from build123d import *

# Parameters (mm, degrees)
SKETCH1_W           = 19
SKETCH1_H           = 25.42
BOSS_EXTRUDE2_DEPTH = 10
FILLET1_R           = 3
SKETCH3_W           = 19.1
SKETCH3_H           = 2.2
CUT_EXTRUDE2_DEPTH  = 115.44
SKETCH4_R           = 9.475
SKETCH4_R_2         = 4.5
SKETCH4_R_3         = 6.33
SKETCH4_R_4         = 3.55
SKETCH4_R_5         = 1.25
CUT_EXTRUDE3_DEPTH  = 11
SKETCH5_W           = 42.44
SKETCH5_H           = 2.2
CUT_EXTRUDE4_DEPTH  = 90.1
SKETCH6_W           = 39.39
SKETCH6_H           = 25.42
CUT_EXTRUDE5_DEPTH  = 3.5
FILLET2_R           = 2
CUT_EXTRUDE6_DEPTH  = 6.5
CUT_EXTRUDE7_DEPTH  = 4.5


with BuildPart() as part:
    # Sketch1 → Boss-Extrude2 (new body)
    with BuildSketch(Plane(origin=(0, 0, 0), x_dir=(1, 0, 0), z_dir=(0, 1, 0))):
        Polygon((54.1, 18.1), (54.1, 0), (22.15, -56.030772795), (-22.15, -56.030772795), (-54.1, 0), (-54.1, 18.89218031), (-15.415468147, 58.409227205), (10.334531853, 58.409227205), align=None)
        with Locations((0, 7.599227205)):
            Rectangle(SKETCH1_W, SKETCH1_H, mode=Mode.SUBTRACT)
    extrude(amount=BOSS_EXTRUDE2_DEPTH)

    # Fillet1
    fillet1_edges = [part.edges().sort_by_distance(p)[0] for p in [
        (-9.5, 5, -20.309227205),
        (-9.5, 5, 5.110772795),
        (9.5, 5, 5.110772795),
        (9.5, 5, -20.309227205),
    ]]
    fillet(fillet1_edges, radius=FILLET1_R)

    # Sketch3 → Cut-Extrude2 (cut, through all)
    with BuildSketch(Plane(origin=(0, 0, -58.409227205), x_dir=(-1, 0, 0), z_dir=(0, 0, -1))):
        with Locations((44.55, 1.1)):
            Rectangle(SKETCH3_W, SKETCH3_H)
    extrude(amount=-CUT_EXTRUDE2_DEPTH, mode=Mode.SUBTRACT)

    # Sketch4 → Cut-Extrude3 (cut, through all)
    with BuildSketch(Plane(origin=(0, 10, 0), x_dir=(1, 0, 0), z_dir=(0, 1, 0))):
        with Locations((-3.065, 45.734227205)):
            Circle(SKETCH4_R)
        with Locations((14.065, -23.816239571)):
            Circle(SKETCH4_R_2)
        with Locations((-5.105, -23.816239571)):
            Circle(SKETCH4_R_2)
        with Locations((4.48, -43.150772795)):
            Circle(SKETCH4_R_2)
        with Locations((38.535, 4.609227205)):
            Circle(SKETCH4_R_3)
        with Locations((14.45, 15.849227205)):
            Circle(SKETCH4_R_4)
        with Locations((14.45, -0.650772795)):
            Circle(SKETCH4_R_4)
        with Locations((-14.45, -0.650772795)):
            Circle(SKETCH4_R_4)
        with Locations((-14.45, 15.849227205)):
            Circle(SKETCH4_R_4)
        with Locations((-50.45, 14.379227205)):
            Circle(SKETCH4_R_5)
    extrude(amount=-CUT_EXTRUDE3_DEPTH, mode=Mode.SUBTRACT)

    # Sketch5 → Cut-Extrude4 (cut, through all)
    with BuildSketch(Plane.ZY.offset(35)):
        with Locations((34.810772795, 1.1)):
            Rectangle(SKETCH5_W, SKETCH5_H)
    extrude(amount=-CUT_EXTRUDE4_DEPTH, mode=Mode.SUBTRACT)

    # Sketch6 → Cut-Extrude5 (cut)
    with BuildSketch(Plane.XZ):
        with Locations((0, -7.599227205)):
            Rectangle(SKETCH6_W, SKETCH6_H)
    extrude(amount=-CUT_EXTRUDE5_DEPTH, mode=Mode.SUBTRACT)

    # Fillet2
    fillet2_edges = [part.edges().sort_by_distance(p)[0] for p in [
        (19.695, 1.75, 5.110772795),
        (19.695, 1.75, -20.309227205),
        (-19.695, 1.75, -20.309227205),
        (-19.695, 1.75, 5.110772795),
    ]]
    fillet(fillet2_edges, radius=FILLET2_R)

    # Sketch4_3 → Cut-Extrude6 (cut)
    with BuildSketch(Plane(origin=(0, 10, 0), x_dir=(1, 0, 0), z_dir=(0, 1, 0))):
        with BuildLine():
            Line((-50, 8.869227205), (-50, 4.289227205))
            ThreePointArc((-50, 4.289227205), (-44.53, -1.180772795), (-39.06, 4.289227205))
            Line((-39.06, 4.289227205), (-39.06, 8.869227205))
            ThreePointArc((-39.06, 8.869227205), (-44.53, 14.339227205), (-50, 8.869227205))
        make_face()
    extrude(amount=-CUT_EXTRUDE6_DEPTH, mode=Mode.SUBTRACT)

    # Sketch7 → Cut-Extrude7 (cut, through all)
    with BuildSketch(Plane(origin=(0, 3.5, 0), x_dir=(-1, 0, 0), z_dir=(0, 1, 0))):
        with BuildLine():
            Line((41.28, -8.869227205), (41.28, -4.289227205))
            ThreePointArc((41.28, -4.289227205), (44.53, -1.039227205), (47.78, -4.289227205))
            Line((47.78, -4.289227205), (47.78, -8.869227205))
            ThreePointArc((47.78, -8.869227205), (44.53, -12.119227205), (41.28, -8.869227205))
        make_face()
    extrude(amount=-CUT_EXTRUDE7_DEPTH, mode=Mode.SUBTRACT)


solid = part.part
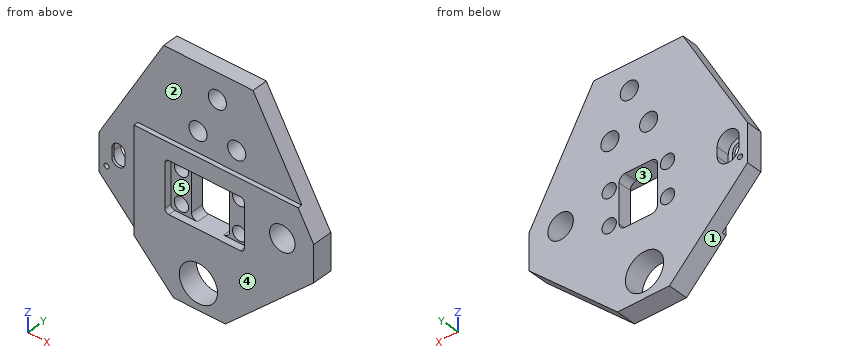
Could you check a few things on this model? Use its own coordinates, in mm. Face numbers are marked on the shaded views. A direction names the side the tool comes from. Round coordinates to 2 decimals unless told otherwise and drop trailing zeros. Write each loop counter-clockwise with the first axis right and the second up, starting at its lowest first coordinate (ties: lowest second). Pieces come first, ordered by that corner, then holes. Notation, with made-up numbers: (44.5, 56.5) -> (74.5, 56.5) arc R26 cw to (74.5, 73.5) -> close; hole circle Ø4 at (75.25, 5.25). An arc over 180 degrees is marked (long way). Use a Markdown table: item, result.
1. Which directions (+Z, -Z, +X, -X, +Y, -Y) give clear straight access to the entire face, cutting with the end or side of a thin tool? Please do the marked faces 4 and 5.
Answer key:
| item | result |
|---|---|
| face 4 | +Z, -Z, +X, -X, -Y |
| face 5 | -Y |
2. Please list where these lines run through material, in increasing order: probe 1 along Z at (x, y) = (-14.45, 6.25); probe 2 along Z at (x, y) = (1, 5.25); probe 3 along Y at (x, z) = (-42.5, -14).
Answer key:
| item | result |
|---|---|
| probe 1 | z = -58.41 to -19.4, -12.3 to -2.9, 4.2 to 56.03 |
| probe 2 | z = -58.41 to -54.29, -37.18 to -20.31, 5.11 to 40.3, 46 to 56.03 |
| probe 3 | y = 2.2 to 10 |
3. If we section it at C-C (x = -44.53): List the corners of the cut face in (y, z) for me, then the cut area to 3 significant figures.
Answer key:
| item | result |
|---|---|
| outline | (2.2, -28.67) -> (10, -28.67) -> (10, -14.34) -> (3.5, -14.34) -> (3.5, -12.12) -> (2.2, -12.12) -> close; (2.2, -1.04) -> (3.5, -1.04) -> (3.5, 1.18) -> (10, 1.18) -> (10, 16.78) -> (2.2, 16.78) -> close |
| area | 239 mm^2 |
4. For pin 1 Ø2 at (y, z) = (2.5, -26.5) entering from +X; pin 2 Ø4 at (x, z) = (-15.5, -9.5) entering from -Y; pin 3 Ø1.1 at (y, z) = (0.5, -0.5) entering from -X; pin 4 Ø14.5 at (x, z) = (4.48, 43.15) entering from +Y, each with a flat end and sliding along its axis, tell me the tip position at first contact or that it passes through.
Answer key:
| item | result |
|---|---|
| pin 1 | stops at x = 46.07 |
| pin 2 | stops at y = 3.5 |
| pin 3 | stops at x = -35 |
| pin 4 | stops at y = 10 |
5. We'd pull the mould along Z, two halves only. Please class the marked faces 1, 2 and 3: +Z half, -Z half, draft (parallel to the pull), parting line (faces both ways), or undercut.
Answer key:
| item | result |
|---|---|
| face 1 | -Z half |
| face 2 | draft |
| face 3 | undercut |
6. If we section it at A-A (x = 12.5): List the corners of the cut face in (y, z) for me.
Answer key:
| item | result |
|---|---|
| outline | (0, -56.41) -> (10, -56.41) -> (10, -18.82) -> (3.5, -18.82) -> (3.5, -20.31) -> (0, -20.31) -> close; (0, 5.11) -> (3.5, 5.11) -> (3.5, 3.62) -> (10, 3.62) -> (10, 19.6) -> (2.2, 19.6) -> (2.2, 13.59) -> (0, 13.59) -> close; (2.2, 28.04) -> (10, 28.04) -> (10, 56.03) -> (2.2, 56.03) -> close; (3.5, -12.88) -> (10, -12.88) -> (10, -2.32) -> (3.5, -2.32) -> close |
7. If we section it at D-D (z = -25.5): List the corners of the cut face in (x, y) for me.
Answer key:
| item | result |
|---|---|
| outline | (-47.63, 2.2) -> (-35, 2.2) -> (-35, 0) -> (46.07, 0) -> (46.07, 10) -> (-47.63, 10) -> close |
8. If we section it at B-B (y = 5): State how many separate pieces and enclosed holes the cut face has, then the cut area to 3 significant figures.
Answer key:
| item | result |
|---|---|
| separate pieces | 1 |
| enclosed holes | 12 |
| area | 7,560 mm^2 |
